from build123d import *

# Parameters (mm, degrees)
SKETCH4_R           = 63.881
BOSS_EXTRUDE1_DEPTH = 169.164
SKETCH5_R           = 63.881
BOSS_EXTRUDE2_DEPTH = 169.164


with BuildPart() as part:
    # Sketch1 → Revolve1 (revolve)
    with BuildSketch(Plane.XY):
        Polygon((-109.982, -63.881), (-59.182, -63.881), (-59.182, -57.0357), (-109.982, -57.3786), align=None)
        Polygon((109.982, -57.3786), (59.182, -57.0357), (59.182, -63.881), (109.982, -63.881), align=None)
    revolve(axis=Axis((-109.982, 0, 0), (1, 0, 0)))



with BuildPart() as body_2:
    # Sketch2 → Revolve2 (revolve)
    with BuildSketch(Plane.XY):
        Polygon((57.3786, 109.982), (57.0357, 59.182), (63.881, 59.182), (63.881, 109.982), align=None)
        Polygon((63.881, -109.982), (57.3786, -109.982), (57.0357, -59.182), (63.881, -59.182), align=None)
    revolve(axis=Axis((0, 0, 0), (0, 1, 0)))


with BuildPart() as part_1:
    add(part.part)

    add(body_2.part)  # Boss-Extrude1 merges body 2
    # Sketch4 → Boss-Extrude1 (add)
    with BuildSketch(Plane(origin=(-59.182, 0, 0), x_dir=(0, 0, -1), z_dir=(1, 0, 0))):
        Circle(SKETCH4_R)
    extrude(amount=BOSS_EXTRUDE1_DEPTH)

    # Sketch5 → Boss-Extrude2 (add)
    with BuildSketch(Plane.XZ.offset(-59.182)):
        Circle(SKETCH5_R)
    extrude(amount=BOSS_EXTRUDE2_DEPTH)

    # Sketch6 → Cut-Revolve1 (revolve, cut)
    with BuildSketch(Plane.XY):
        Polygon((-109.982, -57.3786), (-59.182, -57.0357), (-59.182, -51.1302), (59.182, -51.1302), (59.182, -57.0357), (109.982, -57.3786), (109.982, 0), (-109.982, 0), align=None)
    revolve(axis=Axis((109.982, 0, 0), (-1, 0, 0)), mode=Mode.SUBTRACT)

    # Sketch7 → Cut-Revolve2 (revolve, cut)
    with BuildSketch(Plane.XY):
        Polygon((57.3786, 109.982), (57.0357, 59.182), (51.1302, 59.182), (51.1302, -59.182), (57.0357, -59.182), (57.3786, -109.982), (0, -109.982), (0, 109.982), align=None)
    revolve(axis=Axis((0, 109.982, 0), (0, -1, 0)), mode=Mode.SUBTRACT)


solid = part_1.part
Design review of the part built by this model. Coordinates are the model's own, in mm. A direction names the side the tool comes from. Round coordinates to 2 decimals unless told otherwise and drop trailing zeros. Write each loop counter-clockwise with the first axis right and the second up, starting at its lowest first coordinate (ties: lowest second). Pieces come first, ordered by that corner, then holes.
Item 1: Draft analysis for pull direction Y (two halves, no side actions). For faces 1 (the cylindrical face through (-42.33, -27.49, 43.11)), 2 (the flat face through (21, -59.182, 47)), 3 (the flat face through (-52.3, 109.982, -24)), state which applies: released by +Y, released by -Y, zero draft, split by the parting line, or undercut.
Item 2: Consider section B-B on y = -90.5. Give the boundary of the cut face in (x, z).
Item 3: Wall thickness on L1, parallel to Z at x = 19.5, y = 0; L2, parallel to Z at x = -34.5, y = 2; L3, parallel to Y at x = -57, z = 46.5: over which ranges is each line inside the solid? List them lowest first.
Item 4: Consider section C-C on x = 83.5. Give the boundary of the cut face in (y, z).
Item 5: For pin 1 Ø9.5 at (y, z) = (-51.5, -3.5) entering from -X; pin 2 Ø16.5 at (y, z) = (-8.5, -37.5) entering from -X; pin 3 Ø1 at (x, y) = (-64.5, -40) entering from +Z; pin 4 Ø10 at (x, z) = (-25.5, -44) entering from +Y, all flat-tipped, find the tip position at first contact; note any pin that passes through.
Item 6: For faces 4 (the cylindrical face through (43.16, -27.49, 43.11)), 5 (the flat face through (59.182, -21, 47)), 6 (the cylindrical face through (-13.85, -67.98, 62.36)), list the 3-axis set-ups (+Z, -Z, +X, -X, +Y, -Y) from which the entire face can be reached by the end or side of a thin tool; tool diameter is ignored.
Item 7: Consider section A-A on z = 45. Count the separate pieces of the cut face and the enclosed holes in it, and give its area (3 significant figures).
Check values:
1. face 1: undercut
1. face 2: released by -Y
1. face 3: released by +Y
2. outline: circle Ø127.76 at (0, 0); hole circle Ø114.49 at (0, 0)
3. L1: z = -63.88 to -51.13, 51.13 to 63.88
3. L2: z = -63.85 to -51.09, 51.09 to 63.85
3. L3: y = -43.8 to -21.26, 21.26 to 43.8
4. outline: circle Ø127.76 at (0, 0); hole circle Ø114.4 at (0, 0)
5. pin 1: stops at x = -59.18
5. pin 2: passes through
5. pin 3: stops at z = 50.2
5. pin 4: stops at y = 59.18
6. face 4: +X, -X
6. face 5: +X
6. face 6: -Y
7. separate pieces: 4
7. enclosed holes: 0
7. area: 8,180 mm2
